Verification items for the finished model (mm, model axes). Coordinates: 2 decimals unless noted, no trailing zeros. Order: outer loops, then holes, each group sorted by start corner. A loop starts at its lowest first (then second) coordinate and runs counter-clockwise, first axis right, second up. Notation, with made-up numbers: (10.5, -3.75) -> (52.5, -3.75) arc R20 ccw to (52.5, 25.25) -> close; hole circle Ø2 at (13, 64). An arc over 180 degrees is marked (long way). Write item = value, one per line. Start each with the question number.
1. Cross-section at C-C on y = 78.5. Record the cut outline in (x, z).
2. Cross-section at A-A on z = -0.7. Record the cut outline in (x, y), plus the area to 3 significant figures.
3. Cross-section at B-B on x = 582. Record the cut outline in (y, z), plus the area to 3 significant figures.
4. Go/stop test with flat-tipped pins: P1, Ø1.5, axis at x = 578.5, z = -1.5, coming from the +Y side; P2, Ø3, axis at x = 585.5, z = 1.5, coming from the -Y side; P3, Ø1, axis at y = 46, z = 0, coming from the +X side. Record where each tip stops, or that it passes through.
5. Thickness scan on line 1 along Y through (x, z) = (600, 0.6); line 2 along X through (y, z) = (71.5, -0.3); line 3 along X through (y, z) = (63, -2.15). Record the ranges inside material, lowest first. Write a range as from..to.
6. Cross-section at D-D on y = 30. Record the cut outline in (x, z).
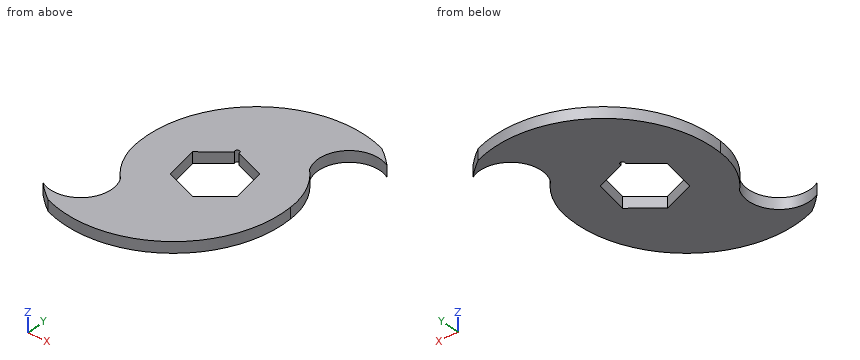
from build123d import *

# Parameters (mm, degrees)
BOSS_EXTRUDE1_DEPTH = 2.5


with BuildPart() as part:
    # Model → Boss-Extrude1 (new, symmetric)
    with BuildSketch(Plane.XY):
        with BuildLine():
            ThreePointArc((625.600029607, 115.214424851), (578.127821467, 108.213195948), (558.208452339, 64.557194238))
            ThreePointArc((558.208452339, 64.557194238), (560.983849767, 52.747710067), (567.839069353, 42.739078209))
            ThreePointArc((567.839069353, 42.739078209), (565.492156458, 25.994108012), (548.747186261, 23.647195117))
            ThreePointArc((548.747186261, 23.647195117), (552.600795358, 20.115585583), (556.747156658, 16.932779125))
            ThreePointArc((556.747156658, 16.932779125), (604.219364798, 23.934008028), (624.138733926, 67.590009739))
            ThreePointArc((624.138733926, 67.590009739), (621.363336499, 79.399493909), (614.508116912, 89.408125767))
            ThreePointArc((614.508116912, 89.408125767), (616.855029807, 106.153095964), (633.600000004, 108.500008859))
            ThreePointArc((633.600000004, 108.500008859), (629.746390907, 112.031618393), (625.600029607, 115.214424851))
        make_face()
        with BuildLine():
            Line((603.1150442, 76.093669174), (589.406378556, 81.08321542))
            ThreePointArc((589.406378556, 81.08321542), (588.293037758, 82.410043316), (587.700641492, 80.782447954))
            Line((587.700641492, 80.782447954), (576.525234868, 71.405168377))
            Line((576.525234868, 71.405168377), (579.232142066, 56.053534802))
            Line((579.232142066, 56.053534802), (593.88050033, 50.721968413))
            Line((593.88050033, 50.721968413), (605.821951397, 60.742035599))
            Line((605.821951397, 60.742035599), (603.1150442, 76.093669174))
        make_face(mode=Mode.SUBTRACT)
    extrude(amount=BOSS_EXTRUDE1_DEPTH, both=True)


solid = part.part
Worked out:
q1.outline = (559.18, -2.5) -> (584.98, -2.5) -> (584.98, 2.5) -> (559.18, 2.5) -> close; (596.5, -2.5) -> (621.74, -2.5) -> (621.74, 2.5) -> (596.5, 2.5) -> close
q2.outline = (548.75, 23.65) arc R60 ccw to (556.75, 16.93) arc R50.21 ccw to (624.14, 67.59) arc R33 ccw to (614.51, 89.41) arc R14.04 cw to (633.6, 108.5) arc R60 ccw to (625.6, 115.21) arc R50.21 ccw to (558.21, 64.56) arc R33 ccw to (567.84, 42.74) arc R14.04 cw to start; hole (576.53, 71.41) -> (579.23, 56.05) -> (593.88, 50.72) -> (605.82, 60.74) -> (603.12, 76.09) -> (589.41, 81.08) arc R1 ccw (long way) to (587.7, 80.78) -> close
q2.area = 4,690 mm²
q3.outline = (14.49, -2.5) -> (55.05, -2.5) -> (55.05, 2.5) -> (14.49, 2.5) -> close; (76, -2.5) -> (110.85, -2.5) -> (110.85, 2.5) -> (76, 2.5) -> close
q3.area = 377 mm²
q4.P1 = 109.03
q4.P2 = 14.85
q4.P3 = 621.09
q5.line_1 = 21.09..55.86, 77.23..117.6
q5.line_2 = 558.2..576.64, 603.93..623.72
q5.line_3 = 558.32..578.01, 605.42..624.25
q6.outline = (568.29, -2.5) -> (610.93, -2.5) -> (610.93, 2.5) -> (568.29, 2.5) -> close
